```python
from build123d import *

# Parameters (mm, degrees)
F0_W     = 1000
F0_H     = 200
F0_R     = 51.5
F1_DEPTH = 18
F0_R_2   = 1.25
F0_R_3   = 66
F0_R_4   = 40
F2_DEPTH = 11


# Not quite as in the source:
# - a feature names something its author has since deleted; it is built from what else it names


with BuildPart() as f1:
    # F0 (on Front) → F1 (new body)
    with BuildSketch(Plane.XZ):
        Rectangle(F0_W, F0_H)
        with BuildLine():
            ThreePointArc((-452.0796354846, 58.0796354846), (-394, 71), (-335.9203645154, 58.0796354846))
            ThreePointArc((-335.9203645154, 58.0796354846), (-323, 0), (-335.9203645154, -58.0796354846))
            ThreePointArc((-335.9203645154, -58.0796354846), (-394, -71), (-452.0796354846, -58.0796354846))
            ThreePointArc((-452.0796354846, -58.0796354846), (-465, 0), (-452.0796354846, 58.0796354846))
        make_face(mode=Mode.SUBTRACT)
        with BuildLine():
            ThreePointArc((-272.0796354846, 58.0796354846), (-214, 71), (-155.9203645154, 58.0796354846))
            ThreePointArc((-155.9203645154, 58.0796354846), (-143, 0), (-155.9203645154, -58.0796354846))
            ThreePointArc((-155.9203645154, -58.0796354846), (-214, -71), (-272.0796354846, -58.0796354846))
            ThreePointArc((-272.0796354846, -58.0796354846), (-285, 0), (-272.0796354846, 58.0796354846))
        make_face(mode=Mode.SUBTRACT)
        Circle(F0_R, mode=Mode.SUBTRACT)
        with BuildLine():
            ThreePointArc((155.9203645154, -58.0796354846), (143, 0), (155.9203645154, 58.0796354846))
            ThreePointArc((155.9203645154, 58.0796354846), (214, 71), (272.0796354846, 58.0796354846))
            ThreePointArc((272.0796354846, 58.0796354846), (285, 0), (272.0796354846, -58.0796354846))
            ThreePointArc((272.0796354846, -58.0796354846), (214, -71), (155.9203645154, -58.0796354846))
        make_face(mode=Mode.SUBTRACT)
        with BuildLine():
            ThreePointArc((335.9203645154, 58.0796354846), (394, 71), (452.0796354846, 58.0796354846))
            ThreePointArc((452.0796354846, 58.0796354846), (465, 0), (452.0796354846, -58.0796354846))
            ThreePointArc((452.0796354846, -58.0796354846), (394, -71), (335.9203645154, -58.0796354846))
            ThreePointArc((335.9203645154, -58.0796354846), (323, 0), (335.9203645154, 58.0796354846))
        make_face(mode=Mode.SUBTRACT)
    extrude(amount=F1_DEPTH)

    # F0 (on Front) → F2 (join)
    with BuildSketch(Plane.XZ):
        with BuildLine():
            ThreePointArc((-335.9203645154, -58.0796354846), (-323, 0), (-335.9203645154, 58.0796354846))
            ThreePointArc((-335.9203645154, 58.0796354846), (-394, 71), (-452.0796354846, 58.0796354846))
            ThreePointArc((-452.0796354846, 58.0796354846), (-465, 0), (-452.0796354846, -58.0796354846))
            ThreePointArc((-452.0796354846, -58.0796354846), (-394, -71), (-335.9203645154, -58.0796354846))
        make_face()
        with Locations((-448.5441015786, -54.5441015786)):
            Circle(F0_R_2, mode=Mode.SUBTRACT)
        with Locations((-339.4558984214, -54.5441015786)):
            Circle(F0_R_2, mode=Mode.SUBTRACT)
        with Locations((-394, 0)):
            Circle(F0_R_3, mode=Mode.SUBTRACT)
        with Locations((-448.5441015786, 54.5441015786)):
            Circle(F0_R_2, mode=Mode.SUBTRACT)
        with Locations((-339.4558984214, 54.5441015786)):
            Circle(F0_R_2, mode=Mode.SUBTRACT)
        with BuildLine():
            ThreePointArc((452.0796354846, -58.0796354846), (465, 0), (452.0796354846, 58.0796354846))
            ThreePointArc((452.0796354846, 58.0796354846), (394, 71), (335.9203645154, 58.0796354846))
            ThreePointArc((335.9203645154, 58.0796354846), (323, 0), (335.9203645154, -58.0796354846))
            ThreePointArc((335.9203645154, -58.0796354846), (394, -71), (452.0796354846, -58.0796354846))
        make_face()
        with Locations((339.4558984214, -54.5441015786)):
            Circle(F0_R_2, mode=Mode.SUBTRACT)
        with Locations((448.5441015786, -54.5441015786)):
            Circle(F0_R_2, mode=Mode.SUBTRACT)
        with Locations((394, 0)):
            Circle(F0_R_3, mode=Mode.SUBTRACT)
        with Locations((339.4558984214, 54.5441015786)):
            Circle(F0_R_2, mode=Mode.SUBTRACT)
        with Locations((448.5441015786, 54.5441015786)):
            Circle(F0_R_2, mode=Mode.SUBTRACT)
        Circle(F0_R)
        with BuildLine():
            ThreePointArc((43.1672658205, 12.7116938911), (44.5394598189, 6.4215667122), (45, 0))
            ThreePointArc((45, 0), (40.3751702485, -19.8707228708), (27.4513054486, -35.6570586163))
            ThreePointArc((27.4513054486, -35.6570586163), (27.6364458273, -36.0112469205), (27.7003363532, -36.4057647469))
            ThreePointArc((27.7003363532, -36.4057647469), (26.8283423835, -37.5972392288), (25.4289580476, -37.1263800096))
            ThreePointArc((25.4289580476, -37.1263800096), (0, -45), (-25.4289580476, -37.1263800096))
            ThreePointArc((-25.4289580476, -37.1263800096), (-27.1850679185, -37.4170359898), (-27.4513054486, -35.6570586163))
            ThreePointArc((-27.4513054486, -35.6570586163), (-42.7975432333, -13.9057647469), (-43.1672658205, 12.7116938911))
            ThreePointArc((-43.1672658205, 12.7116938911), (-43.9863638787, 14.2920359898), (-42.3947978504, 15.0891058459))
            ThreePointArc((-42.3947978504, 15.0891058459), (-26.4503363532, 36.4057647469), (-1.2498794309, 44.9826388889))
            ThreePointArc((-1.2498794309, 44.9826388889), (-0.0086807649, 46.2499698574), (1.25, 45))
            ThreePointArc((1.25, 45), (1.2499698574, 44.9913192351), (1.2498794309, 44.9826388889))
            ThreePointArc((1.2498794309, 44.9826388889), (26.4503363532, 36.4057647469), (42.3947978504, 15.0891058459))
            ThreePointArc((42.3947978504, 15.0891058459), (43.5252341949, 14.9221140295), (44.0475432333, 13.9057647469))
            ThreePointArc((44.0475432333, 13.9057647469), (43.8036876648, 13.1640280126), (43.1672658205, 12.7116938911))
        make_face(mode=Mode.SUBTRACT)
        with BuildLine():
            ThreePointArc((27.4513054486, -35.6570586163), (40.3751702485, -19.8707228708), (45, 0))
            ThreePointArc((45, 0), (44.5394598189, 6.4215667122), (43.1672658205, 12.7116938911))
            ThreePointArc((43.1672658205, 12.7116938911), (41.6087225879, 13.5194935039), (42.3947978504, 15.0891058459))
            ThreePointArc((42.3947978504, 15.0891058459), (26.4503363532, 36.4057647469), (1.2498794309, 44.9826388889))
            ThreePointArc((1.2498794309, 44.9826388889), (0, 43.75), (-1.2498794309, 44.9826388889))
            ThreePointArc((-1.2498794309, 44.9826388889), (-26.4503363532, 36.4057647469), (-42.3947978504, 15.0891058459))
            ThreePointArc((-42.3947978504, 15.0891058459), (-41.7811939506, 14.6334557085), (-41.5475432333, 13.9057647469))
            ThreePointArc((-41.5475432333, 13.9057647469), (-42.055806499, 12.8996203154), (-43.1672658205, 12.7116938911))
            ThreePointArc((-43.1672658205, 12.7116938911), (-42.7975432333, -13.9057647469), (-27.4513054486, -35.6570586163))
            ThreePointArc((-27.4513054486, -35.6570586163), (-26.0558185268, -35.2196552727), (-25.2003363532, -36.4057647469))
            ThreePointArc((-25.2003363532, -36.4057647469), (-25.2588618713, -36.7837707772), (-25.4289580476, -37.1263800096))
            ThreePointArc((-25.4289580476, -37.1263800096), (0, -45), (25.4289580476, -37.1263800096))
            ThreePointArc((25.4289580476, -37.1263800096), (25.7156047878, -35.3944935039), (27.4513054486, -35.6570586163))
        make_face()
        Circle(F0_R_4, mode=Mode.SUBTRACT)
    extrude(amount=F2_DEPTH)


solid = f1.part
```
CAD build for the part. Positions are in the model's coordinates, mm. A direction names the side the tool comes from. Give positions to 0.01 mm unless a question says otherwise; leave off trailing zeros. Order: outer loops, then holes, each group sorted by start corner. A loop starts at its lowest first (then second) coordinate and runs counter-clockwise, first axis right, second up.
(1) Flat gauge pin, fed straight in: pin 1 (4 mm diameter, centred on x = -448.54, z = -54.54, fed in from -Y). Where does the tip first touch, or does it go through?
(2) Saw through at C-C, the plane x = -189.5. Give the cut face in (y, z).
(3) Saw through at A-A, the plane x = -394. Give the cut face in (y, z).
(4) Mould opens along X. For faces 4 (the flat face through (-426, -11, 58)), 5 (the cylindrical face through (-8.67, -5.42, -39.05)), 6 (the flat face through (-7, -9, -100)), 7 (the flat face through (-500, -9, -1)) say: released by +X, released by -X, zero draft, split by the parting line, or undercut.
(5) Tool access for faces 1 (the flat face through (-7, -18, -65)), 2 (the cylindrical face through (284.997, -8.874, 0.84)), 3 (the flat face through (30.3, -11, -26.5)): list every direction of +Z, -Z, +X, -X, +Y, -Y with a clear straight run to the whole face (end or side of a thin tool).
(6) Drill centre lines: L1, parallel to Z at x = -394, y = -3; L2, parallel to X at y = -8.75, z = -42; L3, parallel to X at y = -5.25, z = 20.5. Where is each one in solid material? Low to high.
(7) Saw through at B-B, the plane z = 0. State how many separate pieces and enclosed holes the cut face has, then the cut area to 4 significant figures.
Results found:
1. pin 1: stops at y = -11
2. outline: (-18, -100) - (0, -100) - (0, -68.79) - (-18, -68.79) - close; (-18, 68.79) - (0, 68.79) - (0, 100) - (-18, 100) - close
3. outline: (-18, -100) - (0, -100) - (0, -66) - (-11, -66) - (-11, -71) - (-18, -71) - close; (-18, 71) - (-11, 71) - (-11, 66) - (0, 66) - (0, 100) - (-18, 100) - close
4. face 4: undercut
4. face 5: undercut
4. face 6: zero draft
4. face 7: released by -X
5. face 1: +Z, -Z, +X, -X, -Y
5. face 2: +Y, -Y
5. face 3: -Y
6. L1: z = -100 to -66, 66 to 100
6. L2: x = -500 to -444.91, -343.09 to -278.4, -149.6 to 149.6, 278.4 to 343.09, 444.91 to 500
6. L3: x = -500 to -456.74, -331.26 to -283.46, -144.54 to -34.35, 34.35 to 144.54, 283.46 to 331.26, 456.74 to 500
7. separate pieces: 6
7. enclosed holes: 0
7. area: 6,395 mm2
